Could you check a few things on this model? Use its own coordinates, in mm. A direction names the side the tool comes from. Give positions to 0.01 mm unless a question says otherwise; leave off trailing zeros. Write each loop counter-clockwise with the first axis right and the second up, starting at its lowest first coordinate (ties: lowest second). Pieces come first, ordered by that corner, then holes. Notation, with made-up numbers: (18.25, 21) - (70.25, 21) arc R12 ccw to (70.25, 33) - close; hole circle Ø11 at (-35, -17.5). An arc over 180 degrees is marked (long way). Answer in a Markdown table with one row per item.
from build123d import *


with BuildPart() as f1:
    # F0 (on Front) → F1 (revolve)
    with BuildSketch(Plane.XZ):
        with BuildLine():
            Line((-26.804441, 0), (0, 0))
            Line((0, 0), (0, 3.5))
            Line((0, 3.5), (-23.311267, 3.5))
            ThreePointArc((-23.311267, 3.5), (-37.439592, 9.344067), (-43.311229, 23.460957))
            Line((-43.311229, 23.460957), (-43.323994, 30))
            Line((-43.323994, 30), (-46.824001, 30))
            Line((-46.824001, 30), (-46.809776, 22.713209))
            Line((-46.809776, 22.713209), (-46.807706, 21.653051))
            Line((-46.807706, 21.653051), (-46.805643, 20.596067))
            Line((-46.805643, 20.596067), (-46.804403, 19.960957))
            ThreePointArc((-46.804403, 19.960957), (-46.802858, 19.748387), (-46.799054, 19.535845))
            ThreePointArc((-46.799054, 19.535845), (-40.78151, 5.694702), (-26.804441, 0))
        make_face()
        Polygon((-48.95586, 22.709019), (-46.807706, 21.653051), (-46.809776, 22.713209), align=None)
        Polygon((-48.95586, 21.653051), (-46.805643, 20.596067), (-46.807706, 21.653051), align=None)
        with BuildLine():
            Line((-48.95586, 20.596067), (-46.799054, 19.535845))
            ThreePointArc((-46.799054, 19.535845), (-46.802858, 19.748387), (-46.804403, 19.960957))
            Line((-46.804403, 19.960957), (-46.805643, 20.596067))
            Line((-46.805643, 20.596067), (-48.95586, 20.596067))
        make_face()
    revolve(axis=Axis((0, 0, 15), (0, 0, 1)))


solid = f1.part
1) Will these pins go through, and if not, where does the flat tip stop? P1, Ø6, axis at y = 30, z = 9, coming from the +X side; P2, Ø10, axis at x = 29.5, z = 4.5, coming from the -Y side; P3, Ø4, axis at y = 33.5, z = 26.5, coming from the +X side.
Check values:
| item | result |
|---|---|
| P1 | stops at x = 34.99 |
| P2 | stops at y = -34.09 |
| P3 | stops at x = 34.64 |
2) Imagine slicing it at B-B (z = 15.5). List the corners of the cut face in (x, y) for me.
Check values:
| item | result |
|---|---|
| outline | circle Ø92.58 at (0, 0); hole circle Ø83.28 at (0, 0) |
3) On a 3-axis mill with a long thin cutter (end or side, diameter ignored), from which of +Z, -Z, +X, -X, +Y, -Y can I reach the whole of each face in a straight line? I mean faces 1 (the face through (40, 25, 21.653)), 2 (the face through (0, 0, 3.5)). Say none if no direction works.
Check values:
| item | result |
|---|---|
| face 1 | none |
| face 2 | +Z |
4) Imagine slicing it at A-A (z = 25.5). List the corners of the cut face in (x, y) for me.
Check values:
| item | result |
|---|---|
| outline | circle Ø93.63 at (0, 0); hole circle Ø86.63 at (0, 0) |
5) If I drill on line 1 (Z direction, x = -7, y = -1); line 2 (Y direction, x = 25, z = 8.5); line 3 (Y direction, x = -20.5, z = 15.5), over which ranges is the centre line in solid material (lowest first)?
Check values:
| item | result |
|---|---|
| line 1 | z = 0 to 3.5 |
| line 2 | y = -35.19 to -26.65, 26.65 to 35.19 |
| line 3 | y = -41.5 to -36.25, 36.25 to 41.5 |
6) We'd pull the mould along Z, two halves only. Please class faces 3 (the face through (10.149, 45.704, 26.306)), 4 (the face through (40, 25, 20.596)), 5 (the face through (0, 0, 0)), 6 (the face through (41.4, 13.7, 30)): +Z half, -Z half, draft (parallel to the pull), parting line (faces both ways), or undercut.
Check values:
| item | result |
|---|---|
| face 3 | undercut |
| face 4 | undercut |
| face 5 | -Z half |
| face 6 | +Z half |
